Verification items for this drawing (mm, ordinates from the low corner). A direction names the side the tool comes from. Round coordinates to 2 decimals unless told otherwise and drop trailing zeros. Order: outer loops, then holes, each group sorted by start corner. A loop starts at its lowest first (then second) coordinate and runs counter-clockwise, first axis right, second up.
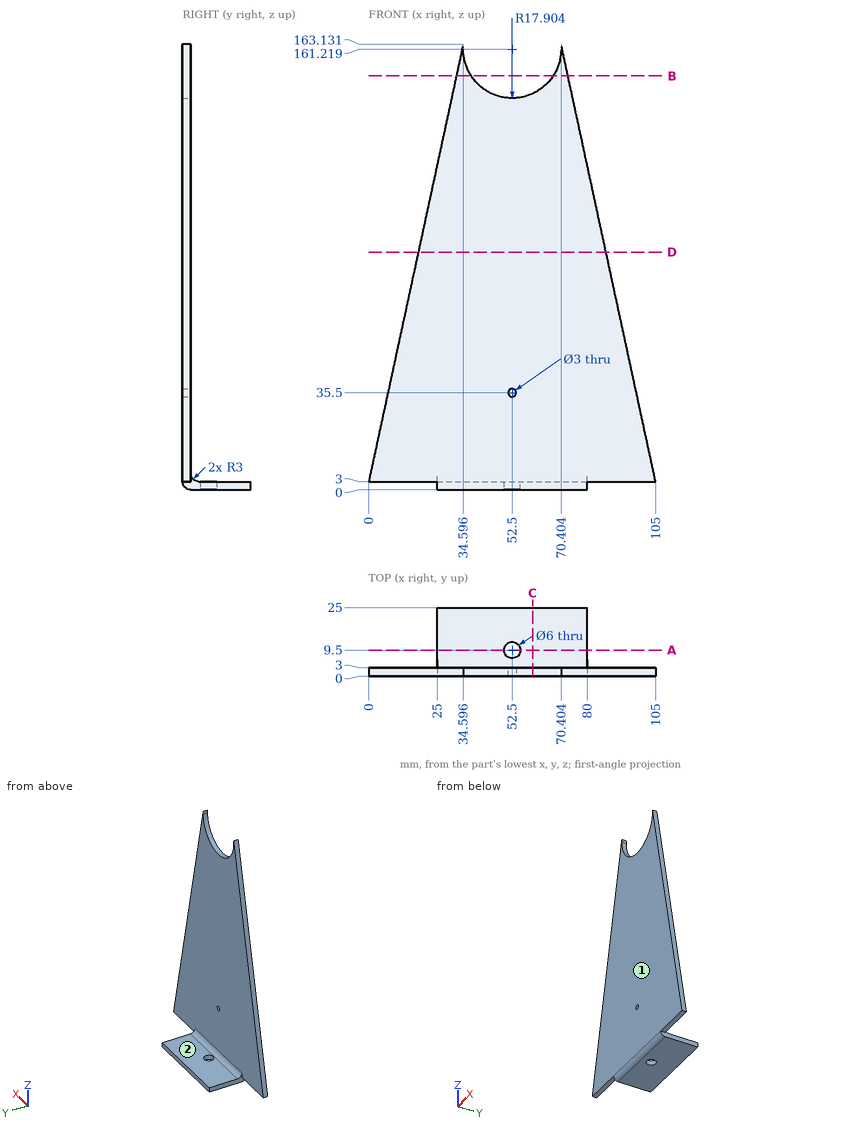
Item 1: Scan lines: line 1 along X through (y, z) = (9.5, 0.8); line 2 along Z through (x, y) = (59.5, 6.25). Record each from-to range of solid material in increasing order.
Answer:
line 1: x = 25 to 49.5, 55.5 to 80
line 2: z = 0 to 3
Item 2: Sectioned sample at C-C (x = 60). Record the cut outline in (y, z).
Answer:
outline: (0, 3) arc R3 ccw to (3, 0) - (25, 0) - (25, 3) - (6, 3) arc R3 cw to (3, 6) - (3, 144.96) - (0, 144.96) - close
Item 3: Sectioned sample at D-D (z = 87). Record the cut outline in (x, y), and give its area (3 significant figures).
Answer:
outline: (18.15, 0) - (86.85, 0) - (86.85, 3) - (18.15, 3) - close
area: 206 mm2
Item 4: Access from +Z, -Z, +X, -X, +Y, -Y to the whole of each face (thin tool, end or side, straight path). Record for the marked faces 1 and 2.
Answer:
face 1: +Z, -Z, +X, -X, -Y
face 2: +Z, +X, -X, +Y
Item 5: Sectioned sample at B-B (z = 151.5). Record the cut outline in (x, y), and give its area (3 significant figures).
Answer:
outline: (32.08, 0) - (37.46, 0) - (37.46, 3) - (32.08, 3) - close; (67.54, 0) - (72.92, 0) - (72.92, 3) - (67.54, 3) - close
area: 32.3 mm2
Item 6: Go/stop test with flat-tipped pins: P1, Ø1, axis at x = 56.5, z = 118, coming from the +Y side; P2, Ø5.5, axis at x = 41.5, y = 11, coming from the +Z side; P3, Ø1, axis at y = 1, z = 162.5, coming from the -X side; P4, Ø2.5, axis at x = 52.5, z = 35.5, coming from the -Y side. Record where each tip stops, or that it passes through.
Answer:
P1: stops at y = 3
P2: stops at z = 3
P3: stops at x = 34.35
P4: passes through
Item 7: Sectioned sample at A-A (y = 9.5). Record the cut outline in (x, z).
Answer:
outline: (25, 0) - (49.5, 0) - (49.5, 3) - (25, 3) - close; (55.5, 0) - (80, 0) - (80, 3) - (55.5, 3) - close
